Solid Edge part; units mm, degrees
sketch "Sketch1" plane through (0, 0, 0) normal (0, 0, 1) x (1, 0, 0)
  circle A0 centre (0, 0) radius 4.35
extrude "Protrusion1" add sketch "Sketch1" along normal blind 6
sketch "Sketch2" plane through (0, 0, 0) normal (0, 0, -1) x (1, 0, 0)
  circle A0 centre (0, 0) radius 5.5081
  circle A1 centre (0, 0) radius 1.5
extrude "Wycięcie_1" cut sketch "Sketch2" against normal blind 1.2
sketch "Sketch3" plane through (0, 0, 1.2) normal (0, 0, -1) x (1, 0, 0)
  circle A0 centre (0, 0) radius 3.85
  circle A1 centre (0, 0) radius 1.5
extrude "Wycięcie_2" cut sketch "Sketch3" against normal blind 4.5
sketch "Sketch4" plane through (0, 0, 1.2) normal (0, 0, -1) x (0, 1, 0)
  circle A0 centre (0, 0) radius 3.25
  circle A1 centre (0, 0) radius 4
extrude "Wyciągnięcie_2" add sketch "Sketch4" against normal blind 1
fillet "Zaokrąglenie_1" radius 1 1 edges at (-4.35, 0, 6)
Source: CAD feature listing. Evaluate the final solid. Frame: model axes, mm. A direction names the side the tool comes from. Round coordinates to 2 decimals unless told otherwise and drop trailing zeros. Loops run counter-clockwise (first coordinate to the right, second up) from the corner with the lowest first, then second, coordinate; pieces in that order, holes last.
1. Contact query for a flat-ended pin moving along its axis: pin 1 (2 mm diameter, centred on x = -3, y = 2, fed in from -Z). Output: stop coordinate, or through.
2. Mould query, pull axis X, two halves, no side actions, for faces 4 (the flat face through (0, 0, 6)), 5 (the flat face through (-2, 0, 5.7)), 6 (the cylindrical face through (-0.943, 4.247, 3.073)), 7 (the cylindrical face through (-0.83, 3.76, 3.93)). Classes: released by +X, released by -X, zero draft, split by the parting line, or undercut.
3. Ray query, L1, parallel to X at y = 0, z = 4; L2, parallel to X at y = 0, z = 1.95. Return the intervals inside material, ascending.
4. Section query D-D on z = 5.5. Output: boundary loops of the cut face in (x, y).
5. Section query C-C on z = 4.25. Output: boundary loops of the cut face in (x, y).
6. Access query for faces 1 (the flat face through (3, -2, 2.2)), 2 (the cylindrical face through (-1.978, -2.579, 1.693)), 3 (the flat face through (0, 0, 0)). Directions: +Z, -Z, +X, -X, +Y, -Y. A direction counts if a zero-diameter tool reaches every point of the face in a straight line with its end or side. Return the directions, or none.
7. Section query A-A on x = 0. Output: boundary loops of the cut face in (y, z), and give its area (3 significant figures).
Answers below:
1. pin 1: stops at z = 1.2
2. face 4: zero draft
2. face 5: undercut
2. face 6: split by the parting line
2. face 7: undercut
3. L1: x = -4.35 to -3.85, -1.5 to 1.5, 3.85 to 4.35
3. L2: x = -4.35 to -3.25, -1.5 to 1.5, 3.25 to 4.35
4. outline: circle Ø8.43 at (0, 0); circle Ø3 at (0, 0); hole circle Ø7.7 at (0, 0)
5. outline: circle Ø8.7 at (0, 0); circle Ø3 at (0, 0); hole circle Ø7.7 at (0, 0)
6. face 1: none
6. face 2: -Z
6. face 3: -Z, +X, -X, +Y, -Y
7. outline: (-4.35, 1.2) - (-3.25, 1.2) - (-3.25, 2.2) - (-3.85, 2.2) - (-3.85, 5.7) - (-1.5, 5.7) - (-1.5, 0) - (1.5, 0) - (1.5, 5.7) - (3.85, 5.7) - (3.85, 2.2) - (3.25, 2.2) - (3.25, 1.2) - (4.35, 1.2) - (4.35, 5) arc R1 ccw to (3.35, 6) - (-3.35, 6) arc R1 ccw to (-4.35, 5) - close
7. area: 25.0 mm2
